Input: part model. Units: mm. Frame: model coordinates. A direction names the side the tool comes from. Coordinates: 2 decimals unless noted, no trailing zeros. Order: outer loops, then holes, each group sorted by start corner. A loop starts at its lowest first (then second) coordinate and runs counter-clockwise, first axis right, second up.
from build123d import *

# Parameters (mm, degrees)
F1_DEPTH  = 20
F3_DEPTH  = 20
F4_R      = 12
F5_R      = 10
F6_DEPTH  = 25
F7_R      = 10
F8_DEPTH  = 25
F9_R      = 9
F10_DEPTH = 25


with BuildPart() as f1:
    # F0 (on Top) → F1 (new body)
    with BuildSketch(Plane.XY):
        Polygon((150, 0), (0, 0), (0, -35), (150, -75), align=None)
    extrude(amount=-F1_DEPTH)

    # F2 (on face) → F3 (join)
    with BuildSketch(Plane(origin=(0, 0, 0), x_dir=(-1, 0, 0), z_dir=(0, 1, 0))):
        Polygon((-150, 40), (-150, 0), (-50, 0), (-50, 60), align=None)
    extrude(amount=-F3_DEPTH)

    # F4
    f4_edges = [f1.edges().sort_by_distance(p)[0] for p in [
        (0, -35, -10),
        (150, -75, -10),
        (50, -10, 60),
        (150, -10, 40),
    ]]
    fillet(f4_edges, radius=F4_R)

    # F5 (on face) → F6 (cut)
    with BuildSketch(Plane.XY):
        with Locations((12, -25.780660243)):
            Circle(F5_R)
    extrude(amount=-F6_DEPTH, mode=Mode.SUBTRACT)

    # F7 (on face) → F8 (cut)
    with BuildSketch(Plane.XY):
        with Locations((138, -59.380660243)):
            Circle(F7_R)
    extrude(amount=-F8_DEPTH, mode=Mode.SUBTRACT)

    # F9 (on face) → F10 (cut)
    with BuildSketch(Plane.XZ.offset(20)):
        with Locations((62, 45.3623531674)):
            Circle(F9_R)
    extrude(amount=-F10_DEPTH, mode=Mode.SUBTRACT)


solid = f1.part
Item 1: Access query for faces 4 (the face through (50, -10, 22)), 5 (the face through (147.237, -63.211, -9.86)), 6 (the face through (101, -20, 23)). Directions: +Z, -Z, +X, -X, +Y, -Y. A direction counts if a zero-diameter tool reaches every point of the face in a straight line with its end or side. Return the directions, or none.
Response values:
face 4: +Z, -X, +Y, -Y
face 5: +Z, -Z
face 6: +Z, +X, -X, -Y
Item 2: Cut plane A-A on x = 138. Return loops of the section in (y, z), then the cut area to 3 significant figures.
Response values:
outline: (-71.38, -20) - (-69.38, -20) - (-69.38, 0) - (-71.38, 0) - close; (-49.38, -20) - (0, -20) - (0, 42.4) - (-20, 42.4) - (-20, 0) - (-49.38, 0) - close
area: 1,880 mm2
Item 3: Cut plane D-D on y = -21.5. Return loops of the section in (x, z), then the cut area to 3 significant figures.
Response values:
outline: (0, -20) - (2.96, -20) - (2.96, 0) - (0, 0) - close; (21.04, -20) - (150, -20) - (150, 0) - (21.04, 0) - close
area: 2,640 mm2
Item 4: Cut plane B-B on z = -10. Return loops of the section in (x, y), then the cut area to 3 significant figures.
Response values:
outline: (0, -25.78) arc R12 ccw to (8.91, -37.38) - (134.91, -70.98) arc R12 ccw to (150, -59.38) - (150, 0) - (0, 0) - close; hole circle Ø20 at (12, -25.78); hole circle Ø20 at (138, -59.38)
area: 7,550 mm2
Item 5: Ray query, probe 1 along Z at (x, y) = (62, -10.5); probe 2 along Z at (x, y) = (70, -42.5); probe 3 along Y at (x, z) = (138, -12.75). Return the intervals inside material, ascending.
Response values:
probe 1: z = -20 to 36.36, 54.36 to 57.36
probe 2: z = -20 to 0
probe 3: y = -71.38 to -69.38, -49.38 to 0
Item 6: Pin query (flat end, axial travel): pin 1 Ø16 at (y, z) = (-11, 17) entering from -X; pin 2 Ø17 at (x, z) = (94.5, 26.5) entering from -Y; pin 3 Ø10 at (x, y) = (81, -31.5) entering from +Z. Return the tip coordinate at first contact, or that it passes through.
Response values:
pin 1: stops at x = 50
pin 2: stops at y = -20
pin 3: stops at z = 0
Item 7: Cut plane C-C on x = 12. Return loops of the section in (y, z).
Response values:
outline: (-38.2, -20) - (-35.78, -20) - (-35.78, 0) - (-38.2, 0) - close; (-15.78, -20) - (0, -20) - (0, 0) - (-15.78, 0) - close
Item 8: Draft query along X for faces 1 (the face through (9.832, -35.543, -9.86)), 2 (the face through (0, -13, -10)), 3 (the face through (93, 0, 11)). Return one class per face: pulls with the +X half, pulls with the -X half, needs draft (parallel to the pull), parting line crosses it, or undercut.
Response values:
face 1: undercut
face 2: pulls with the -X half
face 3: needs draft
